Could you check a few things on this model? Use its own coordinates, in mm. A direction names the side the tool comes from. Coordinates: 2 decimals unless noted, no trailing zeros. Write each loop counter-clockwise with the first axis right and the second up, starting at its lowest first coordinate (ties: lowest second). Pieces come first, ordered by that corner, then holes. Notation, with made-up numbers: (-14, 89) - (8, 89) arc R29 ccw to (8, 114) - close; hole circle Ø7 at (8, 22). An arc over 180 degrees is marked (long way). Answer as a JSON object with one key per item and string values. Group by question number.
1) If we section it at D-D (x = 20): Write out the boundary of the cut face in (y, z), plus the area to 3 significant figures.
2) Will these pins go through, and if not, where does the flat tip stop? pin 1 Ø18 at (x, z) = (-20, 20) entering from -Y; pin 2 Ø3 at (x, z) = (-24.5, 27) entering from +Y; pin 3 Ø6 at (y, z) = (-16, -20.5) entering from -X.
3) If we section it at B-B (x = 0): Write out the boundary of the cut face in (y, z), plus the area to 3 significant figures.
4) If we section it at C-C (z = 12.5): Write out the boundary of the cut face in (x, y), plus the area to 3 significant figures.
5) We'd pull the mould along Z, two halves only. Please class faces 1 (the cylindrical face through (-49.01, 10.46, -17)), 2 (the flat face through (8, -8, -50)), 3 (the cylindrical face through (0.56, 46.99, 47.15)), 4 (the cylindrical face through (-29.54, 49.01, -17)): released by +Z, released by -Z, zero draft, split by the parting line, or undercut.
6) Please list where these lines run through material, in increasing order: line 1 along X through (y, z) = (-21, 18); line 2 along Y through (x, z) = (-13, -16); line 3 along Z through (x, y) = (-48.95, -20).
7) On a 3-axis mill with a long thin cutter (end or side, diameter ignored), from which of +Z, -Z, +X, -X, +Y, -Y can I reach the whole of each face in a straight line? I mean faces 5 (the flat face through (48, 20, 0)), 6 (the cylindrical face through (-49.01, -29.54, 23)), 7 (the cylindrical face through (10.46, 49.01, -17)). Say none if no direction works.
```python
from build123d import *

# Parameters (mm, degrees)
F0_W      = 100
F0_H      = 100
F1_DEPTH  = 50
F2_R      = 10
F3_R      = 10
F4_DEPTH  = 2
F5_R      = 10
F6_DEPTH  = 2
F7_R      = 10
F8_DEPTH  = 2
F9_R      = 10
F10_DEPTH = 2
F11_R     = 10
F12_DEPTH = 2
F13_R     = 10
F14_DEPTH = 2


with BuildPart() as f1:
    # F0 (on Top) → F1 (new body, symmetric)
    with BuildSketch(Plane.XY):
        Rectangle(F0_W, F0_H)
    extrude(amount=F1_DEPTH, both=True)

    # F2
    f2_edges = [f1.edges().sort_by_distance(p)[0] for p in [
        (50, 50, 0),
        (-50, -50, 0),
        (50, -50, 0),
        (0, -50, -50),
        (0, -50, 50),
        (50, 0, -50),
        (50, 0, 50),
        (-50, 0, 50),
        (-50, 50, 0),
        (0, 50, -50),
        (0, 50, 50),
        (-50, 0, -50),
    ]]
    fillet(f2_edges, radius=F2_R)

    # F3 (on face) → F4 (cut)
    with BuildSketch(Plane.XY.offset(50)):
        Circle(F3_R)
    extrude(amount=-F4_DEPTH, mode=Mode.SUBTRACT)

    # F5 (on face) → F6 (cut)
    with BuildSketch(Plane.XZ.offset(50)):
        with Locations((-20, 20)):
            Circle(F5_R)
        with Locations((20, -20)):
            Circle(F5_R)
    extrude(amount=-F6_DEPTH, mode=Mode.SUBTRACT)

    # F7 (on face) → F8 (cut)
    with BuildSketch(Plane(origin=(0, 0, -50), x_dir=(1, 0, 0), z_dir=(0, 0, -1))):
        with Locations((-20, 20)):
            Circle(F7_R)
        Circle(F7_R)
        with Locations((20, -20)):
            Circle(F7_R)
    extrude(amount=-F8_DEPTH, mode=Mode.SUBTRACT)

    # F9 (on face) → F10 (cut)
    with BuildSketch(Plane(origin=(0, 50, 0), x_dir=(-1, 0, 0), z_dir=(0, 1, 0))):
        with Locations((-20, 20)):
            Circle(F9_R)
        with Locations((20, 20)):
            Circle(F9_R)
        with Locations((20, -20)):
            Circle(F9_R)
        with Locations((-20, -20)):
            Circle(F9_R)
    extrude(amount=-F10_DEPTH, mode=Mode.SUBTRACT)

    # F11 (on face) → F12 (cut)
    with BuildSketch(Plane(origin=(-50, 0, 0), x_dir=(0, -1, 0), z_dir=(-1, 0, 0))):
        Circle(F11_R)
        with Locations((-20, 20)):
            Circle(F11_R)
        with Locations((20, 20)):
            Circle(F11_R)
        with Locations((20, -20)):
            Circle(F11_R)
        with Locations((-20, -20)):
            Circle(F11_R)
    extrude(amount=-F12_DEPTH, mode=Mode.SUBTRACT)

    # F13 (on face) → F14 (cut)
    with BuildSketch(Plane.YZ.offset(50)):
        with Locations((-20, 25)):
            Circle(F13_R)
        with Locations((-20, 0)):
            Circle(F13_R)
        with Locations((-20, -25)):
            Circle(F13_R)
        with Locations((20, -25)):
            Circle(F13_R)
        with Locations((20, 0)):
            Circle(F13_R)
        with Locations((20, 25)):
            Circle(F13_R)
    extrude(amount=-F14_DEPTH, mode=Mode.SUBTRACT)


solid = f1.part
```
Here are the results:
{
 "1": {"outline": "(-50, -40) arc R10 ccw to (-40, -50) - (10, -50) - (10, -48) - (30, -48) - (30, -50) - (40, -50) arc R10 ccw to (50, -40) - (50, -30) - (48, -30) - (48, -10) - (50, -10) - (50, 10) - (48, 10) - (48, 30) - (50, 30) - (50, 40) arc R10 ccw to (40, 50) - (-40, 50) arc R10 ccw to (-50, 40) - (-50, -10) - (-48, -10) - (-48, -30) - (-50, -30) - close", "area": "9,750 mm²"},
 "2": {"pin 1": "stops at y = -48", "pin 2": "stops at y = 48", "pin 3": "stops at x = -48"},
 "3": {"outline": "(-50, -40) arc R10 ccw to (-40, -50) - (-10, -50) - (-10, -48) - (10, -48) - (10, -50) - (40, -50) arc R10 ccw to (50, -40) - (50, 40) arc R10 ccw to (40, 50) - (10, 50) - (10, 48) - (-10, 48) - (-10, 50) - (-40, 50) arc R10 ccw to (-50, 40) - close", "area": "9,830 mm²"},
 "4": {"outline": "(-50, -40) arc R10 ccw to (-40, -50) - (-26.61, -50) - (-26.61, -48) - (-13.39, -48) - (-13.39, -50) - (40, -50) arc R10 ccw to (50, -40) - (50, 40) arc R10 ccw to (40, 50) - (26.61, 50) - (26.61, 48) - (13.39, 48) - (13.39, 50) - (-13.39, 50) - (-13.39, 48) - (-26.61, 48) - (-26.61, 50) - (-40, 50) arc R10 ccw to (-50, 40) - (-50, 26.61) - (-48, 26.61) - (-48, 13.39) - (-50, 13.39) - (-50, -13.39) - (-48, -13.39) - (-48, -26.61) - (-50, -26.61) - close", "area": "9,780 mm²"},
 "5": {"face 1": "undercut", "face 2": "released by -Z", "face 3": "released by +Z", "face 4": "undercut"},
 "6": {"line 1": "x = -48 to 48", "line 2": "y = -50 to 48", "line 3": "z = -44.46 to -30, -10 to 10, 30 to 44.46"},
 "7": {"face 5": "+X", "face 6": "-X", "face 7": "+Y"}
}
